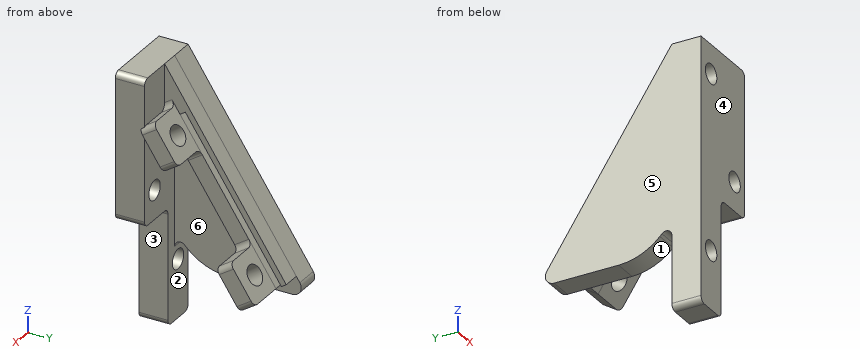
```python
from build123d import *

# Parameters (mm, degrees)
EXTRUDE_1_DEPTH                = 5
EXTRUDE_3_DEPTH                = 4
EXTRUDE_4_DEPTH                = 3
CUT_EXTRUDE_1_DEPTH            = 2
SKETCH_6_R                     = 1.7
CUT_EXTRUDE_1_2_DEPTH          = 5.5
EXTRUDE_5_DEPTH                = 6.5
FILLET_1_R                     = 1
CUT_EXTRUDE_2_REACH            = 56.175
SKETCH_8_R                     = 1.7
FILLET_2_R                     = 1
PATTERN_LINEAR_2_COUNT         = 2
PATTERN_LINEAR_2_PITCH         = 24
FILLET_1_OF_PATTERN_LINEAR_2_R = 1
FILLET_2_OF_PATTERN_LINEAR_2_R = 1
FILLET_3_R                     = 1
FILLET_4_R                     = 1


with BuildPart() as part:
    # 草图1 → 凸台-拉伸1 (new body)
    with BuildSketch(Plane(origin=(0, 0, 0), x_dir=(1, 0, 0), z_dir=(0, 1, 0))):
        with BuildLine():
            Line((0, 0), (0, 44))
            ThreePointArc((0, 44), (0.292893219, 44.707106781), (1, 45))
            Line((1, 45), (5, 45))
            ThreePointArc((5, 45), (5.707106781, 44.707106781), (6, 44))
            Line((6, 44), (6, 26))
            ThreePointArc((6, 26), (6.292893219, 25.292893219), (7, 25))
            Line((7, 25), (12, 25))
            ThreePointArc((12, 25), (12.707106781, 24.707106781), (13, 24))
            Line((13, 24), (13, 1))
            ThreePointArc((13, 1), (12.707106781, 0.292893219), (12, 0))
            Line((12, 0), (0, 0))
        make_face()
    extrude(amount=EXTRUDE_1_DEPTH)

    # 草图3 → 凸台-拉伸3 (add)
    with BuildSketch(Plane(origin=(0, 0, 0), x_dir=(0, 0, -1), z_dir=(1, 0, 0))):
        with BuildLine():
            Line((30, 5), (0, 5))
            Line((0, 5), (32.676465773, 26.464426075))
            ThreePointArc((32.676465773, 26.464426075), (34.212284585, 26.53080998), (35, 25.210715033))
            Line((35, 25.210715033), (35, 14.142135624))
            ThreePointArc((35, 14.142135624), (34.238795325, 10.3153013), (32.071067812, 7.071067812))
            Line((32.071067812, 7.071067812), (30, 5))
        make_face()
    extrude(amount=EXTRUDE_3_DEPTH)

    # 草图4 → 凸台-拉伸4 (add)
    with BuildSketch(Plane(origin=(4, 0, 0), x_dir=(0, 0, -1), z_dir=(1, 0, 0))):
        Polygon((0, 5), (31.760679732, 25.862867084), (34.505793822, 21.683830277), (9.107089607, 5), align=None)
    extrude(amount=EXTRUDE_4_DEPTH)

    # 草图5 → Cut-Extrude 1 (cut)
    with BuildSketch(Plane(origin=(7, 0, 0), x_dir=(0, 0, -1), z_dir=(1, 0, 0))):
        Polygon((32.30970255, 25.027059723), (7.235481709, 8.556375183), (7.839406809, 7.636987085), (32.91362765, 24.107671625), align=None)
    extrude(amount=-CUT_EXTRUDE_1_DEPTH, mode=Mode.SUBTRACT)

    # 草图6 → Cut-Extrude 1 2 (cut)
    with BuildSketch(Plane.XZ):
        with Locations(Location((3, -5, 0), (0, 0, 270))):
            Circle(SKETCH_6_R)
        with Locations(Location((3, -35, 0), (0, 0, 270))):
            Circle(SKETCH_6_R)
        with Locations(Location((10, -20, 0), (0, 0, 270))):
            Circle(SKETCH_6_R)
    extrude(amount=-CUT_EXTRUDE_1_2_DEPTH, mode=Mode.SUBTRACT)

    # 草图7 → 凸台-拉伸5 (add)
    with BuildSketch(Plane(origin=(7, 0, 0), x_dir=(0, 0, -1), z_dir=(1, 0, 0))):
        Polygon((32.91362765, 24.107671625), (34.505793822, 21.683830277), (28.237238612, 17.566159142), (26.64507244, 19.99000049), align=None)
    extrude_5 = extrude(amount=EXTRUDE_5_DEPTH)

    # 圆角1
    fillet_1_edges = [part.edges().sort_by_distance(p)[0] for p in [
        (13.5, 18.778079816, -27.441155526),
        (13.5, 22.895750951, -33.709710736),
    ]]
    fillet(fillet_1_edges, radius=FILLET_1_R)

    # 草图8 → 切除-拉伸2 (cut, up to next)
    with BuildSketch(Plane(origin=(0, 1.737674268, 1.141438646), x_dir=(1, 0, 0), z_dir=(0, 0.8358073613682734, 0.549022817998127)), mode=Mode.PRIVATE) as cut_extrude_2_sk1:
        with Locations(Location((9.8, 37.04511409, 0), (0, 0, 270))):
            Circle(SKETCH_8_R)
    cut_extrude_2_tool1 = extrude(cut_extrude_2_sk1.sketch, amount=-CUT_EXTRUDE_2_REACH, mode=Mode.PRIVATE) & part.part
    cut_extrude_2 = cut_extrude_2_tool1.solids().sort_by_distance((9.8, 22.076287, -29.82114))[0]
    add(cut_extrude_2, mode=Mode.SUBTRACT)

    # 圆角2
    fillet_2_edges = [part.edges().sort_by_distance(p)[0] for p in [
        (7, 18.778079816, -27.441155526),
    ]]
    fillet(fillet_2_edges, radius=FILLET_2_R)

    # 阵列(线性)2: 凸台-拉伸5, 切除-拉伸2 ×2
    with Locations(*[Vector(0, -0.549022817998128, 0.8358073613682727) * (i * PATTERN_LINEAR_2_PITCH) for i in range(1, PATTERN_LINEAR_2_COUNT)]):
        add(extrude_5)
        add(cut_extrude_2, mode=Mode.SUBTRACT)

    # 圆角1 of 阵列(线性)2
    fillet_1_of_pattern_linear_2_edges = [part.edges().sort_by_distance(p)[0] for p in [
        (13.5, 5.601532184, -7.381778853),
        (13.5, 9.719203319, -13.650334063),
    ]]
    fillet(fillet_1_of_pattern_linear_2_edges, radius=FILLET_1_OF_PATTERN_LINEAR_2_R)

    # 圆角2 of 阵列(线性)2
    fillet_2_of_pattern_linear_2_edges = [part.edges().sort_by_distance(p)[0] for p in [
        (7, 5.601532184, -7.381778853),
    ]]
    fillet(fillet_2_of_pattern_linear_2_edges, radius=FILLET_2_OF_PATTERN_LINEAR_2_R)

    # 圆角3
    fillet_3_edges = [part.edges().sort_by_distance(p)[0] for p in [
        (7, 9.719203319, -13.650334063),
    ]]
    fillet(fillet_3_edges, radius=FILLET_3_R)

    # 圆角4
    fillet_4_edges = [part.edges().sort_by_distance(p)[0] for p in [
        (2, 5, -30),
    ]]
    fillet(fillet_4_edges, radius=FILLET_4_R)


solid = part.part
```
Verification items for the finished model (mm, model axes). Face numbers are marked on the shaded views. A direction names the side the tool comes from. Give positions to 0.01 mm unless a question says otherwise; leave off trailing zeros. Loops run counter-clockwise (first coordinate to the right, second up) from the corner with the lowest first, then second, coordinate; pieces in that order, holes last.
1. Thickness scan on line 1 (X direction, y = 4.1, z = -5); line 2 (X direction, y = 3.75, z = -20); line 3 (Z direction, x = 3.5, y = 1.75). Record the ranges inside material, lowest first.
2. Section check A-A, the plane x = 3. Enter the section's corners in (y, z), then the cut area to 3 significant figures.
3. Mould release check, pull along Y, two halves, no side actions. Record for the marked faces 4, 5 and 6: released by +Y, released by -Y, zero draft, split by the parting line, or undercut.
4. Section check D-D, the plane z = -5. Enter the section's corners in (x, y).
5. Go/stop test with flat-tipped pins: pin 1 Ø2.5 at (x, z) = (3, -5) entering from -Y; pin 2 Ø6 at (x, z) = (2.5, -4.5) entering from +Y; pin 3 Ø5.5 at (x, y) = (9.5, 2) entering from -Z. Record where each tip stops, or that it passes through.
6. Section check B-B, the plane x = 11. Enter the section's corners in (y, z).
7. Section check C-C, the plane z = -38.5. Enter the section's corners in (x, y), then the cut area to 3 significant figures.
8. Set-up check for the marked faces 1, 2 and 3: record each of +Z, -Z, +X, -X, +Y, -Y from which the full face is reachable in a straight line by a thin tool's end or side.
Geometry says:
1. line 1: x = 0 to 1.3, 4.7 to 13
1. line 2: x = 0 to 8.3, 11.7 to 13
1. line 3: z = -45 to -36.62, -33.38 to -6.62, -3.38 to 0
2. outline: (0, -45) - (5, -45) - (5, -36.7) - (0, -36.7) - close; (0, -33.3) - (5, -33.3) - (5, -32.41) arc R1 cw to (6.71, -31.71) - (7.07, -32.07) arc R10 ccw to (14.14, -35) - (25.21, -35) arc R1.5 ccw to (26.46, -32.68) - (5, 0) - (0, 0) - (0, -3.3) - (5.5, -3.3) - (5.5, -6.7) - (0, -6.7) - close
2. area: 576 mm2
3. face 4: released by -Y
3. face 5: zero draft
3. face 6: undercut
4. outline: (0, 0) - (1.3, 0) - (1.3, 5.5) - (4.7, 5.5) - (4.7, 0) - (13, 0) - (13, 5) - (7, 5) - (7, 8.28) - (0, 8.28) - close
5. pin 1: stops at y = 5.5
5. pin 2: stops at y = 9.93
5. pin 3: stops at z = -25.03
6. outline: (0, -25) - (5, -25) - (5, -21.37) - (0, -21.37) - close; (0, -18.63) - (5, -18.63) - (5, -9.11) - (5.81, -10.35) - (8.24, -8.76) - (6.81, -6.59) - (5, -7.78) - (5, 0) - (0, 0) - close; (7.14, -12.36) - (8.51, -14.45) - (10.93, -12.85) - (9.56, -10.77) - close; (17.57, -28.24) - (18.99, -30.41) - (21.42, -28.81) - (19.99, -26.65) - close; (20.31, -32.42) - (21.68, -34.51) - (24.11, -32.91) - (22.74, -30.83) - close
7. outline: (0, 0) - (6, 0) - (6, 5) - (0, 5) - close
7. area: 30.0 mm2
8. face 1: -Z, +X, -X
8. face 2: -Z, +X
8. face 3: -Z, +X, -Y
